Verification items for the finished model (mm, model axes). A direction names the side the tool comes from. Give positions to 0.01 mm unless a question says otherwise; leave off trailing zeros. Write each loop counter-clockwise with the first axis right and the second up, starting at its lowest first coordinate (ties: lowest second). Pieces come first, ordered by that corner, then holes. Notation, with made-up numbers: (-14, 37.5) -> (40, 37.5) arc R24 cw to (40, 65.5) -> close; hole circle Ø6 at (66.5, 42). An arc over 180 degrees is marked (long way). Answer as CSV lines item,"result".
```python
from build123d import *

# Parameters (mm, degrees)
SKETCH1_W           = 18
SKETCH1_H           = 139.694434203
BOSS_EXTRUDE1_DEPTH = 3
SKETCH4_W           = 3.2
SKETCH4_H           = 10.2
SKETCH4_W_2         = 5.2
SKETCH4_H_2         = 3.2
CUT_EXTRUDE2_DEPTH  = 4


with BuildPart() as part:
    # Sketch1 → Boss-Extrude1 (new body)
    with BuildSketch(Plane(origin=(0, 0, 0), x_dir=(1, 0, 0), z_dir=(0, 1, 0))):
        with Locations((0, -69.847217102)):
            Rectangle(SKETCH1_W, SKETCH1_H)
    extrude(amount=-BOSS_EXTRUDE1_DEPTH)

    # Sketch4 → Cut-Extrude2 (cut, through all)
    with BuildSketch(Plane(origin=(0, 0, 0), x_dir=(1, 0, 0), z_dir=(0, 1, 0))):
        Polygon((5.9, -19.794434203), (9.1, -19.794434203), (9.1, 0.1), (2.4, 0.1), (2.4, -3.1), (5.9, -3.1), align=None)
        with Locations((7.5, -54.694434203)):
            Rectangle(SKETCH4_W, SKETCH4_H)
        with Locations((7.5, -34.694434203)):
            Rectangle(SKETCH4_W, SKETCH4_H)
        with Locations((7.5, -134.694434203)):
            Rectangle(SKETCH4_W, SKETCH4_H)
        with Locations((7.5, -114.694434203)):
            Rectangle(SKETCH4_W, SKETCH4_H)
        with Locations((-7.5, -54.694434203)):
            Rectangle(SKETCH4_W, SKETCH4_H)
        with Locations((-7.5, -114.694434203)):
            Rectangle(SKETCH4_W, SKETCH4_H)
        with Locations((-7.5, -74.694434203)):
            Rectangle(SKETCH4_W, SKETCH4_H)
        with Locations((-7.5, -134.694434203)):
            Rectangle(SKETCH4_W, SKETCH4_H)
        with Locations((-7.5, -34.694434203)):
            Rectangle(SKETCH4_W, SKETCH4_H)
        with Locations((-7.5, -94.694434203)):
            Rectangle(SKETCH4_W, SKETCH4_H)
        Polygon((5.9, -83.644434203), (-0.1, -83.644434203), (-0.1, -86.844434203), (5.9, -86.844434203), (5.9, -99.794434203), (9.1, -99.794434203), (9.1, -69.594434203), (5.9, -69.594434203), align=None)
        with Locations((0, -138.194434203)):
            Rectangle(SKETCH4_W_2, SKETCH4_H_2)
        Polygon((-9.1, 0.1), (-9.1, -19.794434203), (-5.9, -19.794434203), (-5.9, -3.1), (-2.4, -3.1), (-2.4, 0.1), align=None)
    extrude(amount=-CUT_EXTRUDE2_DEPTH, mode=Mode.SUBTRACT)


solid = part.part
```
1) Draft check along Z on faces 6 (the flat face through (0, -3, 69)), 7 (the flat face through (7, -1, 129.594)), 8 (the flat face through (3, -1, 83.644)). Enter one of: +Z half, -Z half, draft (parallel to the pull), parting line (faces both ways), or undercut.
Reported:
face 6,"draft"
face 7,"+Z half"
face 8,"undercut"
2) Scan lines: line 1 along Z through (x, y) = (6, -2); line 2 along Z through (x, y) = (1.75, -2.6); line 3 along Z through (x, y) = (3.5, -1.95). Record each from-to range of solid material in increasing order.
Reported:
line 1,"19.79 to 29.59, 39.79 to 49.59, 59.79 to 69.59, 99.79 to 109.59, 119.79 to 129.59"
line 2,"0 to 83.64, 86.84 to 136.59"
line 3,"3.1 to 83.64, 86.84 to 139.69"
3) Section check B-B (z = 74). Record the boundary of the cut face in (x, y).
Reported:
outline,"(-5.9, -3) -> (5.9, -3) -> (5.9, 0) -> (-5.9, 0) -> close"
4) Section check A-A (x = 7.25). Record the boundary of the cut face in (y, z).
Reported:
outline,"(-3, 19.79) -> (0, 19.79) -> (0, 29.59) -> (-3, 29.59) -> close; (-3, 39.79) -> (0, 39.79) -> (0, 49.59) -> (-3, 49.59) -> close; (-3, 59.79) -> (0, 59.79) -> (0, 69.59) -> (-3, 69.59) -> close; (-3, 99.79) -> (0, 99.79) -> (0, 109.59) -> (-3, 109.59) -> close; (-3, 119.79) -> (0, 119.79) -> (0, 129.59) -> (-3, 129.59) -> close"
5) Depth check by flat-ended pin: pin 1 (1.5 mm diameter, centred on y = -1, z = 114, fed in from +X); pin 2 (0.9 mm diameter, centred on x = -7, y = -1, fed in from -Z); pin 3 (0.9 mm diameter, centred on y = -1, z = 115, fed in from -X). Enter the tip coordinate at first touch or a pass-through.
Reported:
pin 1,"x = 5.9"
pin 2,"z = 19.79"
pin 3,"x = -5.9"
6) Tool access check on faces 1 (the flat face through (-0.1, -1, 85)), 2 (the flat face through (2.4, -1, 2)), 3 (the flat face through (5.9, -1, 135)), 4 (the flat face through (-5.9, -1, 135)), 5 (the flat face through (-7, -1, 79.794)). Record the directions out of +Z, -Z, +X, -X, +Y, -Y that give a thin tool (end or side, any length) a straight path to the whole face; none if there is none.
Reported:
face 1,"+X, +Y, -Y"
face 2,"-Z, +X, +Y, -Y"
face 3,"+Z, +X, +Y, -Y"
face 4,"+Z, -X, +Y, -Y"
face 5,"-X, +Y, -Y"
